Source: three-view drawing plus pictorial views. Frame: mm from the lowest corner of the part. Coordinates: 2 decimals unless noted, no trailing zeros. Loops run counter-clockwise (first coordinate to the right, second up) from the corner with the lowest first, then second, coordinate; pieces in that order, holes last. Notation, with made-up numbers: M 65,87 L 114,87 A13 cw 114,94 Z; hole C 61.5,41.25 d6. An arc over 180 degrees is marked long. Use a Markdown table: item, result. Add a question column.
1. Section C-C on x = 15.75. Output: boundary loops of the cut face in (y, z), then the cut area to 3 significant figures.
2. Pin query (flat end, axial travel): pin 1 (5 mm diameter, centred on y = 3, z = 10, fed in from +X). Return the tip coordinate at first contact, or that it passes through.
3. Section D-D on z = 42. Output: boundary loops of the cut face in (x, y).
4. Section B-B on y = 2.5. Output: boundary loops of the cut face in (x, z).
5. Section A-A on x = 12.5. Output: boundary loops of the cut face in (y, z), then the cut area to 3 significant figures.
6. Draft query along Z for the marked faces 1, 2, 3 and 4. Return one class per face: +Z half, -Z half, draft (parallel to the pull), parting line (faces both ways), or undercut.
7. Line query: L1, parallel to Z at x = 12.5, y = 24; L2, parallel to X at y = 16, z = 54; L3, parallel to Z at x = 11.5, y = 19 (1 decimal). Output: solid intervals per line, ascending. Write a range as [from, to].
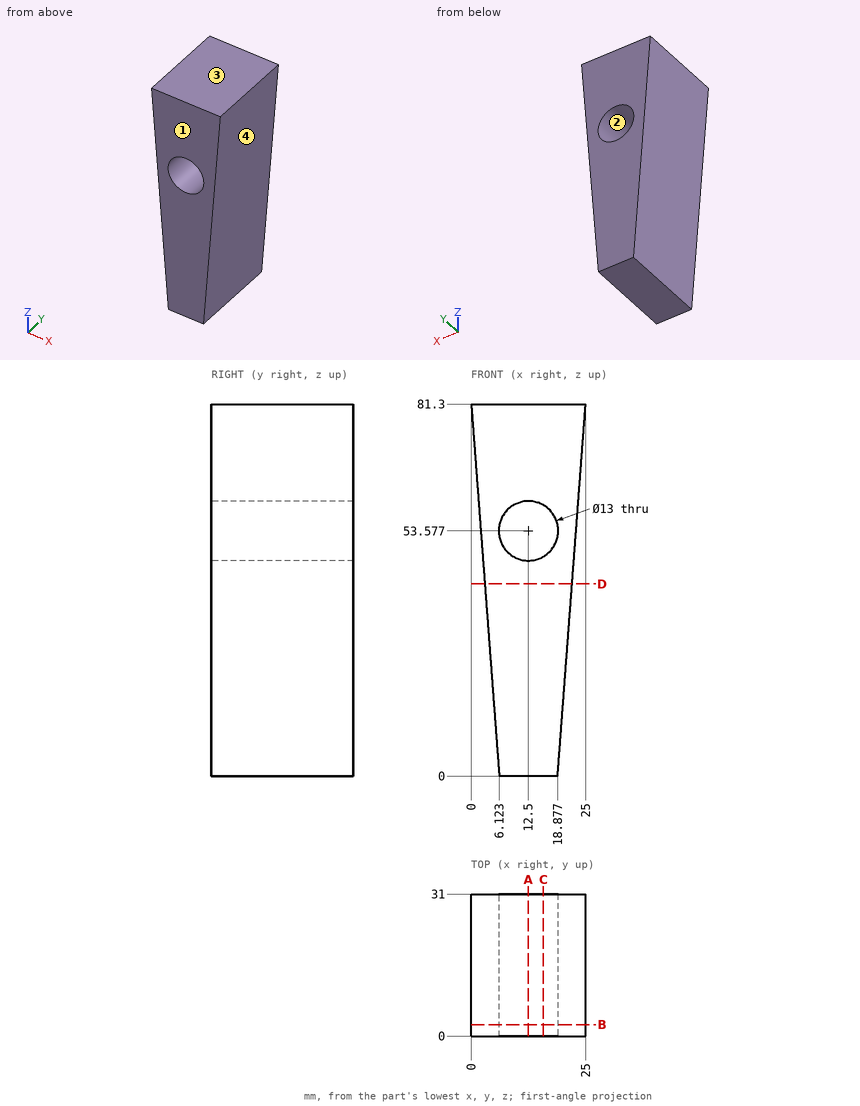
Answers below:
| question | item | result |
|---|---|---|
| 1 | outline | M 0,0 L 31,0 L 31,47.95 L 0,47.95 Z; M 0,59.21 L 31,59.21 L 31,81.3 L 0,81.3 Z |
| 1 | area | 2,170 mm² |
| 2 | pin 1 | stops at x = 19.82 |
| 3 | outline | M 2.96,0 L 22.04,0 L 22.04,31 L 2.96,31 Z |
| 4 | outline | M 0,81.3 L 6.12,0 L 18.88,0 L 25,81.3 Z; hole C 12.5,53.58 d13 |
| 5 | outline | M 0,0 L 31,0 L 31,47.08 L 0,47.08 Z; M 0,60.08 L 31,60.08 L 31,81.3 L 0,81.3 Z |
| 5 | area | 2,120 mm² |
| 6 | face 1 | draft |
| 6 | face 2 | undercut |
| 6 | face 3 | +Z half |
| 6 | face 4 | -Z half |
| 7 | L1 | z = [0, 47.08], [60.08, 81.3] |
| 7 | L2 | x = [2.06, 6.01], [18.99, 22.94] |
| 7 | L3 | z = [0, 47.2], [60, 81.3] |
